Can you work these out from the model? Positions are in its coordinate system, mm. Round coordinates to 2 decimals unless told otherwise and drop trailing zeros. Loops run counter-clockwise (first coordinate to the right, second up) from the corner with the lowest first, then second, coordinate; pieces in that order, holes last. Notation, with made-up numbers: (63.25, -38.75) -> (117.25, -38.75) arc R23 ccw to (117.25, -6.75) -> close; hole circle Ø8 at (41.5, 89). An arc over 180 degrees is marked (long way). Write each question's results on one line, items separated by ' | '.
from build123d import *

# Parameters (mm, degrees)
F3_T     = -3.81
F4_R     = 7.62
F5_DEPTH = 33.02


with BuildPart() as f1:
    # F0 (on Top) → F1 (revolve)
    with BuildSketch(Plane.XY):
        Polygon((0, 152.4), (0, 0), (101.6, 0), align=None)
    revolve(axis=Axis((0, 76.2, 0), (0, 1, 0)))

    # F3
    f3_openings = [f1.faces().sort_by_distance(p)[0] for p in [
        (0, 0, 0),
    ]]
    offset(amount=F3_T, openings=f3_openings)

    # F4 (on offset) → F5 (cut)
    with BuildSketch(Plane.XZ.offset(-152.4)):
        Circle(F4_R)
    extrude(amount=F5_DEPTH, mode=Mode.SUBTRACT)


solid = f1.part
1. If we section it at B-B (x = 0): List the corners of the cut face in (y, z) for me.
Final values:
outline: (0, -101.6) -> (140.97, -7.62) -> (134.1, -7.62) -> (0, -97.02) -> close; (0, 97.02) -> (134.1, 7.62) -> (140.97, 7.62) -> (0, 101.6) -> close
2. Will these pins go through, and if not, where does the flat tip stop? pin 1 (5 mm diameter, centred on x = 72.5, z = 19, fed in from -Y); pin 2 (3 mm diameter, centred on y = 20.5, z = 9, fed in from +X); pin 3 (8 mm diameter, centred on x = 28.5, z = -63, fed in from -Y).
Final values:
pin 1: y = 29.36 | pin 2: x = 88.49 | pin 3: y = 35.81
3. If we section it at D-D (y = 80): List the corners of the cut face in (x, z) for me, then the cut area to 3 significant figures.
Final values:
outline: circle Ø96.53 at (0, 0); hole circle Ø87.38 at (0, 0) | area: 1,320 mm2
4. Please list where these lines run through material, in increasing order: line 1 (Z direction, x = -43.5, y = 74.5); line 2 (Z direction, x = 58.5, y = 11); line 3 (X direction, y = 138.75, z = 0). Write a range as from..to.
Final values:
line 1: -28.37..-18.71, 18.71..28.37 | line 2: -73.92..-67.98, 67.98..73.92 | line 3: -9.1..-7.62, 7.62..9.1
5. If we section it at A-A (z = 0): List the corners of the cut face in (x, y) for me.
Final values:
outline: (-101.6, 0) -> (-97.02, 0) -> (-7.62, 134.1) -> (-7.62, 140.97) -> close; (7.62, 134.1) -> (97.02, 0) -> (101.6, 0) -> (7.62, 140.97) -> close
6. If we section it at C-C (y = 61): List the corners of the cut face in (x, z) for me, then the cut area to 3 significant figures.
Final values:
outline: circle Ø121.87 at (0, 0); hole circle Ø112.71 at (0, 0) | area: 1,690 mm2
7. We'd pull the mould along Z, two halves only. Please class faces 1 (the face through (15.259, 102.798, 29.337)), 2 (the face through (-1.65, 137.58, -7.44)), 3 (the face through (-90, 0, 37)): pulls with the +Z half, pulls with the -Z half, needs draft (parallel to the pull), parting line crosses it, or undercut.
Final values:
face 1: parting line crosses it | face 2: undercut | face 3: needs draft
